Geometry check sheet. Reference: the model listing, model coordinates, mm. Round coordinates to 2 decimals unless told otherwise and drop trailing zeros. Write each loop counter-clockwise with the first axis right and the second up, starting at its lowest first coordinate (ties: lowest second). Pieces come first, ordered by that corner, then holes. Notation, with made-up numbers: (-32, -28.5) -> (5, -28.5) arc R14 ccw to (5, -4.5) -> close; hole circle Ø4 at (44.5, -38). An arc over 180 degrees is marked (long way). Put each result on its own line as item: value. Start each with the question number.
Autodesk Fusion 360 part; units mm, degrees
sketch "Sketch1" plane through (0, 0, 0) normal (0, 0, 1) x (1, 0, 0)
  circle A0 centre (0, 0) radius 50
  circle A1 centre (0, 0) radius 3.25
  line L0 (1.7058, 2.7664) -> (-1.7058, 2.7664)
  dimension "d1" = 100
  dimension "d2" = 6.5
extrude "Extrude1" add sketch "Sketch1" along normal blind 10 contours A0 | A1 L0 | A1 L0
extrude "Extrude2" cut sketch "Sketch1" along normal blind 7 contours A1 L0 picked at (-0.2955, 2.8865)
sketch "Sketch2" plane through (0, 0, 0) normal (0, 1, 0) x (1, 0, 0)
  line L0 (0, 20) -> (0, -60)
  line L1 (30, 20) -> (30, -40.4129)
  line L2 (110, 20) -> (110, -69.665)
  line L3 (-75, 0) -> (110, 0)
  line L4 (-75, -60) -> (115, -60)
  line L5 (90, -50) -> (130, -50)
  circle A0 centre (65.0107, -68.6839) radius 45
  circle A1 centre (65.0107, -68.6839) radius 5
  line L6 (88.6327, -92.3059) -> (41.3887, -92.3059)
  line L7 (41.3887, -92.3059) -> (41.3887, -45.0619)
  line L8 (41.3887, -45.0619) -> (88.6327, -45.0619)
  line L9 (88.6327, -45.0619) -> (88.6327, -92.3059)
  line L10 (88.6327, -92.3059) -> (41.3887, -45.0619) construction
  line L11 (41.3887, -92.3059) -> (88.6327, -45.0619) construction
  circle A2 centre (41.3887, -45.0619) radius 3.5
  circle A3 centre (88.6327, -45.0619) radius 3.5
  circle A4 centre (41.3887, -92.3059) radius 3.5
  circle A5 centre (88.6327, -92.3059) radius 3.5
  line L12 (110, -30) -> (70, 0)
  point P0 (65.0107, -68.6839)
  dimension "d7" = 30
  dimension "d8" = 80
  dimension "d9" = 60
  dimension "d10" = 50
  dimension "d11" = 90
  dimension "d12" = 10
  dimension "d13" = 47.244
  dimension "d14" = 47.244
  dimension "d15" = 7
  dimension "d16" = 7
  dimension "d17" = 7
  dimension "d18" = 7
extrude "Extrude3" add sketch "Sketch2" along normal mid plane 10 contours L1 L2 L3 L5 A0 L12 | L4 A0 L7 L8 L9 A2 A3 | L2 L4 A0 L6 L7 L9 A4 A5 | L4 L7 L8 L9 A2 A3 | L4 L6 L7 L9 A4 A5 | L2 L4 L5 A0 | L2 L4 A0
extrude "Extrude4" add sketch "Sketch1" against normal blind 4
component "6627T54_Stepper Motor (2)" placed x (1, 0, 0) y (0, 0, -1) z (0, 1, 0) at (-34.4133, -232.4903, 46.7909)
(1) Sectioned sample at C-C (y = 30). Record the cut outline in (x, z).
(2) Go/stop test with flat-tipped pins: pin 1 Ø11 at (x, z) = (88.63, 45.06) entering from +Y; pin 2 Ø2.5 at (x, z) = (0, 2) entering from +Y; pin 3 Ø5 at (y, z) = (1.5, 25.5) entering from -X; pin 4 Ø5 at (x, y) = (0.5, -1.5) entering from -Z. Record where each tip stops, or that it passes through.
(3) Material ranges on L1, parallel to Y at x = 88, z = 20.5; L2, parallel to Z at x = 11, y = -17.5; L3, parallel to Y at x = 0, z = 4, recorded low to high. Write a range as from..to.
(4) Mould release check, pull along X, two halves, no side actions. Record for faces 1 (the flat face through (60, 0, 0)), 2 (the flat face through (0, 0, 0)), 3 (the flat face through (30, 0, 25)): +X half, -X half, draft (parallel to the pull), parting line (faces both ways), or undercut.
(5) Sectioned sample at A-A (y = 0). Record the cut outline in (x, z) (3 decimals), and give its area (3 significant figures).
(6) Sectioned sample at B-B (z = 12). Record the cut outline in (x, y).
Found:
1. outline: (-40, -4) -> (40, -4) -> (40, 10) -> (-40, 10) -> close
2. pin 1: y = 5
2. pin 2: y = 50
2. pin 3: x = 30
2. pin 4: z = -4
3. L1: -5..5
3. L2: -4..10
3. L3: -50..2.77, 3.25..50
4. face 1: draft
4. face 2: undercut
4. face 3: -X half
5. outline: (-50, -4) -> (-3.25, -4) -> (-3.25, 0) -> (3.25, 0) -> (3.25, -4) -> (50, -4) -> (50, 0) -> (70, 0) -> (110, 30) -> (110, 69.665) arc R45 ccw (long way) to (30, 40.413) -> (30, 10) -> (-50, 10) -> close; hole circle Ø7 at (41.389, 45.062); hole circle Ø7 at (41.389, 92.306); hole circle Ø10 at (65.011, 68.684); hole circle Ø7 at (88.633, 45.062); hole circle Ø7 at (88.633, 92.306)
5. area: 9,210 mm2
6. outline: (30, -5) -> (86, -5) -> (86, 5) -> (30, 5) -> close
